Here's how the part is built. I have some questions about the finished solid (model axes, mm). Coordinates: 2 decimals unless noted, no trailing zeros. Loops run counter-clockwise (first coordinate to the right, second up) from the corner with the lowest first, then second, coordinate; pieces in that order, holes last.
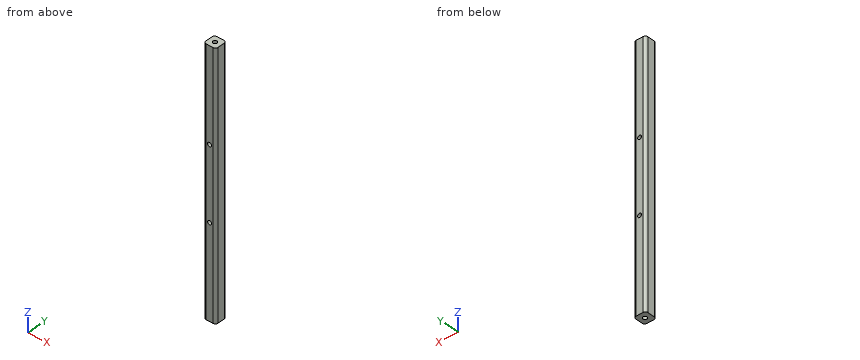
from build123d import *

# Parameters (mm, degrees)
ESQUISSE1_W           = 10
ESQUISSE1_H           = 10
BOSS_EXTRU_1_DEPTH    = 106
TROU_TARAUD_M41_D     = 3.3
TROU_TARAUD_M41_DEPTH = 11.5
TROU_TARAUD_M41_TIP   = 0.991420021
TROU_TARAUD_M42_D     = 3.3
TROU_TARAUD_M42_DEPTH = 11.5
TROU_TARAUD_M42_TIP   = 0.991420021
CONG_1_R              = 2
TROU_TARAUD_M44_D     = 3.3


with BuildPart() as part:
    # Esquisse1 → Boss.-Extru.1 (new, symmetric)
    with BuildSketch(Plane.XY):
        Rectangle(ESQUISSE1_W, ESQUISSE1_H)
    extrude(amount=BOSS_EXTRU_1_DEPTH, both=True)

    # Trou taraudé M41
    with Locations(Plane.XY.offset(106)):
        with Locations((0, 0)):
            Hole(TROU_TARAUD_M41_D / 2, depth=TROU_TARAUD_M41_DEPTH)
            with Locations((0, 0, -(TROU_TARAUD_M41_DEPTH + TROU_TARAUD_M41_TIP / 2))):  # 118° drill point
                Cone(0, TROU_TARAUD_M41_D / 2, TROU_TARAUD_M41_TIP, mode=Mode.SUBTRACT)

    # Trou taraudé M42
    with Locations(Plane(origin=(0, 0, -106), x_dir=(-1, 0, 0), z_dir=(0, 0, -1))):
        with Locations((0, 0)):
            Hole(TROU_TARAUD_M42_D / 2, depth=TROU_TARAUD_M42_DEPTH)
            with Locations((0, 0, -(TROU_TARAUD_M42_DEPTH + TROU_TARAUD_M42_TIP / 2))):  # 118° drill point
                Cone(0, TROU_TARAUD_M42_D / 2, TROU_TARAUD_M42_TIP, mode=Mode.SUBTRACT)

    # Congé1
    cong_1_edges = [part.edges().sort_by_distance(p)[0] for p in [
        (-5, 5, 0),
        (5, 5, 0),
        (5, -5, 0),
        (-5, -5, 0),
    ]]
    fillet(cong_1_edges, radius=CONG_1_R)

    # Trou taraudé M44 (through all)
    with Locations(Plane(origin=(0, 5, 0), x_dir=(1, 0, 0), z_dir=(0, 1, 0))):
        with Locations((0, -30), (0, 30)):
            Hole(TROU_TARAUD_M44_D / 2)


solid = part.part
Q1. Suppose I cut it at A-A on z = -75.5. Write out the boundary of the cut face in (x, y).
Q2. Please list where these lines run through material, in increasing order: probe 1 along Z at (x, y) = (0, 2); probe 2 along X at (y, z) = (2.5, 30); probe 3 along Z at (x, y) = (0.75, 2).
Q3. Will this pin go through, and if not, where does the flat tip stop? P1, Ø2, axis at x = 0, y = 0, coming from the -Z side.
Check values:
1. outline: (-5, -3) arc R2 ccw to (-3, -5) - (3, -5) arc R2 ccw to (5, -3) - (5, 3) arc R2 ccw to (3, 5) - (-3, 5) arc R2 ccw to (-5, 3) - close
2. probe 1: z = -106 to -31.65, -28.35 to 28.35, 31.65 to 106
2. probe 2: x = -5 to -1.65, 1.65 to 5
2. probe 3: z = -106 to -31.47, -28.53 to 28.53, 31.47 to 106
3. P1: stops at z = -94.11
